Here's how the part is built. I have some questions about the finished solid (model axes, mm). A direction names the side the tool comes from. Give positions to 0.01 mm unless a question says otherwise; leave off trailing zeros. Write each loop counter-clockwise with the first axis right and the second up, starting at its lowest first coordinate (ties: lowest second). Pieces come first, ordered by that corner, then holes. Notation, with made-up numbers: (-11, 16) -> (33, 16) arc R25 ccw to (33, 44) -> close; hole circle Ø5 at (-20, 83). An arc over 180 degrees is marked (long way). Use one line per item in the form item = value.
```python
from build123d import *

# Parameters (mm, degrees)
BOSS_EXTRU_1_DEPTH       = 6
ESQUISSE4_W              = 107.5
ESQUISSE4_H              = 70
ENL_V_MAT_EXTRU_3_DEPTH  = 6
CONG_1_R                 = 20
CONG_2_R                 = 8
CONG_3_R                 = 3
ESQUISSE7_W              = 15
ESQUISSE7_H              = 3
ENL_V_MAT_EXTRU_6_DEPTH  = 10
ESQUISSE6_R              = 2
ENL_V_MAT_EXTRU_5_DEPTH  = 10
ESQUISSE8_R              = 2
ESQUISSE8_W              = 6
ESQUISSE8_H              = 12
ENL_V_MAT_EXTRU_7_DEPTH  = 10
ESQUISSE9_R              = 2
ESQUISSE9_W              = 6
ESQUISSE9_H              = 6
ENL_V_MAT_EXTRU_8_DEPTH  = 10
ESQUISSE10_W             = 15
ESQUISSE10_H             = 3
ENL_V_MAT_EXTRU_9_DEPTH  = 10
ESQUISSE11_R             = 1.5
ESQUISSE11_R_2           = 2
ESQUISSE11_R_3           = 1
ESQUISSE11_W             = 10
ESQUISSE11_H             = 6
ENL_V_MAT_EXTRU_10_DEPTH = 10


with BuildPart() as part:
    # Esquisse1 → Boss.-Extru.1 (new body)
    with BuildSketch(Plane(origin=(0, 0, 0), x_dir=(1, 0, 0), z_dir=(0, 1, 0))):
        with BuildLine():
            Line((-159.651418776, 61.996478628), (-151.00295557, 16.28223991))
            ThreePointArc((-151.00295557, 16.28223991), (-144.111724845, 4.599428553), (-131.351536794, 0))
            Line((-131.351536794, 0), (-50.176822125, 0))
            ThreePointArc((-50.176822125, 0), (0, -8.568957982), (50.176822125, 0))
            Line((50.176822125, 0), (131.351536794, 0))
            ThreePointArc((131.351536794, 0), (144.111724845, 4.599428553), (151.00295557, 16.28223991))
            Line((151.00295557, 16.28223991), (159.651418776, 61.996478628))
            ThreePointArc((159.651418776, 61.996478628), (159.912664005, 63.847205713), (160, 65.714238717))
            Line((160, 65.714238717), (160, 154.285761283))
            ThreePointArc((160, 154.285761283), (158.521020838, 161.833727042), (154.30282129, 168.265364394))
            Line((154.30282129, 168.265364394), (109.621642599, 213.979603112))
            ThreePointArc((109.621642599, 213.979603112), (103.077942966, 218.433557202), (95.31882131, 220))
            Line((95.31882131, 220), (-95.31882131, 220))
            ThreePointArc((-95.31882131, 220), (-103.077942966, 218.433557202), (-109.621642599, 213.979603112))
            Line((-109.621642599, 213.979603112), (-154.30282129, 168.265364394))
            ThreePointArc((-154.30282129, 168.265364394), (-158.521020838, 161.833727042), (-160, 154.285761283))
            Line((-160, 154.285761283), (-160, 65.714238717))
            ThreePointArc((-160, 65.714238717), (-159.912664005, 63.847205713), (-159.651418776, 61.996478628))
        make_face()
    extrude(amount=BOSS_EXTRU_1_DEPTH)

    # Esquisse4 → Enlèv. mat.-Extru.3 (cut)
    with BuildSketch(Plane(origin=(0, 6, 0), x_dir=(1, 0, 0), z_dir=(0, 1, 0))):
        with Locations((-98.75, 31)):
            Rectangle(ESQUISSE4_W, ESQUISSE4_H)
        with Locations((98.75, 31)):
            Rectangle(ESQUISSE4_W, ESQUISSE4_H)
    extrude(amount=-ENL_V_MAT_EXTRU_3_DEPTH, mode=Mode.SUBTRACT)

    # Congé1
    cong_1_edges = [part.edges().sort_by_distance(p)[0] for p in [
        (-45, 3, 1.716975434),
        (45, 3, 1.716975434),
    ]]
    fillet(cong_1_edges, radius=CONG_1_R)

    # Congé2
    cong_2_edges = [part.edges().sort_by_distance(p)[0] for p in [
        (-45, 3, -66),
        (-152.5, 3, -66),
        (152.5, 3, -66),
        (45, 3, -66),
    ]]
    fillet(cong_2_edges, radius=CONG_2_R)

    # Congé3
    cong_3_edges = [part.edges().sort_by_distance(p)[0] for p in [
        (-152.5, 3, -24.195350576),
        (152.5, 3, -24.195350576),
    ]]
    fillet(cong_3_edges, radius=CONG_3_R)

    # Esquisse7 → Enlèv. mat.-Extru.6 (cut)
    with BuildSketch(Plane(origin=(0, 6, 0), x_dir=(1, 0, 0), z_dir=(0, 1, 0))):
        with Locations((-25, 67.499999998)):
            Rectangle(ESQUISSE7_W, ESQUISSE7_H)
        with Locations((25, 67.499999998)):
            Rectangle(ESQUISSE7_W, ESQUISSE7_H)
    extrude(amount=-ENL_V_MAT_EXTRU_6_DEPTH, mode=Mode.SUBTRACT)

    # Esquisse6 → Enlèv. mat.-Extru.5 (cut)
    with BuildSketch(Plane(origin=(0, 6, 0), x_dir=(1, 0, 0), z_dir=(0, 1, 0))):
        with Locations(Location((0, 210, 0), (0, 0, 270))):
            Circle(ESQUISSE6_R)
    extrude(amount=-ENL_V_MAT_EXTRU_5_DEPTH, mode=Mode.SUBTRACT)

    # Esquisse8 → Enlèv. mat.-Extru.7 (cut)
    with BuildSketch(Plane(origin=(0, 6, 0), x_dir=(1, 0, 0), z_dir=(0, 1, 0))):
        with Locations(Location((-89.9, 110, 0), (0, 0, 270))):
            Circle(ESQUISSE8_R)
        with Locations(Location((-68.76, 110, 0), (0, 0, 270))):
            Circle(ESQUISSE8_R)
        with Locations(Location((-41.76, 110, 0), (0, 0, 270))):
            Circle(ESQUISSE8_R)
        with Locations(Location((41.76, 110, 0), (0, 0, 270))):
            Circle(ESQUISSE8_R)
        with Locations(Location((68.76, 110, 0), (0, 0, 270))):
            Circle(ESQUISSE8_R)
        with Locations(Location((89.9, 110, 0), (0, 0, 270))):
            Circle(ESQUISSE8_R)
        with Locations((-89.9, 96)):
            Rectangle(ESQUISSE8_W, ESQUISSE8_H)
        with Locations((-89.9, 124)):
            Rectangle(ESQUISSE8_W, ESQUISSE8_H)
        with Locations((-68.76, 96)):
            Rectangle(ESQUISSE8_W, ESQUISSE8_H)
        with Locations((-68.76, 124)):
            Rectangle(ESQUISSE8_W, ESQUISSE8_H)
        with Locations((-41.76, 96)):
            Rectangle(ESQUISSE8_W, ESQUISSE8_H)
        with Locations((-41.76, 124)):
            Rectangle(ESQUISSE8_W, ESQUISSE8_H)
        with Locations((41.76, 96)):
            Rectangle(ESQUISSE8_W, ESQUISSE8_H)
        with Locations((41.76, 124)):
            Rectangle(ESQUISSE8_W, ESQUISSE8_H)
        with Locations((68.76, 96)):
            Rectangle(ESQUISSE8_W, ESQUISSE8_H)
        with Locations((68.76, 124)):
            Rectangle(ESQUISSE8_W, ESQUISSE8_H)
        with Locations((89.9, 96)):
            Rectangle(ESQUISSE8_W, ESQUISSE8_H)
        with Locations((89.9, 124)):
            Rectangle(ESQUISSE8_W, ESQUISSE8_H)
    extrude(amount=-ENL_V_MAT_EXTRU_7_DEPTH, mode=Mode.SUBTRACT)

    # Esquisse9 → Enlèv. mat.-Extru.8 (cut)
    with BuildSketch(Plane(origin=(0, 6, 0), x_dir=(1, 0, 0), z_dir=(0, 1, 0))):
        with Locations(Location((147, 118.4, 0), (0, 0, 270))):
            Circle(ESQUISSE9_R)
        with Locations(Location((147, 87.4, 0), (0, 0, 270))):
            Circle(ESQUISSE9_R)
        with Locations((154, 118.4)):
            Rectangle(ESQUISSE9_W, ESQUISSE9_H)
        with Locations((154, 87.4)):
            Rectangle(ESQUISSE9_W, ESQUISSE9_H)
        with Locations((140, 118.4)):
            Rectangle(ESQUISSE9_W, ESQUISSE9_H)
        with Locations((140, 87.4)):
            Rectangle(ESQUISSE9_W, ESQUISSE9_H)
    extrude(amount=-ENL_V_MAT_EXTRU_8_DEPTH, mode=Mode.SUBTRACT)

    # Esquisse10 → Enlèv. mat.-Extru.9 (cut)
    with BuildSketch(Plane(origin=(0, 6, 0), x_dir=(1, 0, 0), z_dir=(0, 1, 0))):
        with Locations((-25, 176.83)):
            Rectangle(ESQUISSE10_W, ESQUISSE10_H)
        with Locations((25, 176.83)):
            Rectangle(ESQUISSE10_W, ESQUISSE10_H)
    extrude(amount=-ENL_V_MAT_EXTRU_9_DEPTH, mode=Mode.SUBTRACT)

    # Esquisse11 → Enlèv. mat.-Extru.10 (cut)
    with BuildSketch(Plane(origin=(0, 6, 0), x_dir=(-1, 0, 0), z_dir=(0, 1, 0))):
        with Locations(Location((40, -23.835046453, 0), (0, 0, 90))):
            Circle(ESQUISSE11_R)
        with Locations(Location((-40, -23.835046453, 0), (0, 0, 90))):
            Circle(ESQUISSE11_R)
        with Locations(Location((100.750206469, -212.903490041, 0), (0, 0, 90))):
            Circle(ESQUISSE11_R)
        with Locations(Location((152.964714587, -159.569337314, 0), (0, 0, 90))):
            Circle(ESQUISSE11_R)
        with Locations(Location((50.375103235, -212.903490041, 0), (0, 0, 90))):
            Circle(ESQUISSE11_R)
        with Locations(Location((-152.964714587, -159.569337314, 0), (0, 0, 90))):
            Circle(ESQUISSE11_R)
        with Locations(Location((-100.750206469, -212.903490041, 0), (0, 0, 90))):
            Circle(ESQUISSE11_R)
        with Locations(Location((-50.375103235, -212.903490041, 0), (0, 0, 90))):
            Circle(ESQUISSE11_R)
        with Locations(Location((0, -44.911042018, 0), (0, 0, 90))):
            Circle(ESQUISSE11_R)
        with Locations(Location((-109.47882131, -189.64, 0), (0, 0, 90))):
            Circle(ESQUISSE11_R_2)
        with Locations(Location((109.47882131, -189.64, 0), (0, 0, 90))):
            Circle(ESQUISSE11_R_2)
        with Locations(Location((142, -99.324238717, 0), (0, 0, 90))):
            Circle(ESQUISSE11_R_3)
        with Locations(Location((126, -99.324238717, 0), (0, 0, 90))):
            Circle(ESQUISSE11_R_3)
        with Locations(Location((126, -115.324238717, 0), (0, 0, 90))):
            Circle(ESQUISSE11_R_3)
        with Locations(Location((142, -115.324238717, 0), (0, 0, 90))):
            Circle(ESQUISSE11_R_3)
        with Locations((155, -130.324238717)):
            Rectangle(ESQUISSE11_W, ESQUISSE11_H)
        with Locations((155, -83.324238717)):
            Rectangle(ESQUISSE11_W, ESQUISSE11_H)
    extrude(amount=-ENL_V_MAT_EXTRU_10_DEPTH, mode=Mode.SUBTRACT)


solid = part.part
```
Q1. I want a section at C-C, the plane x = 125. Write out the boundary of the cut face in (y, z), and give its area (3 significant figures).
Result set:
outline = (0, -198.25) -> (6, -198.25) -> (6, -66) -> (0, -66) -> close
area = 793 mm2
Q2. I want a section at A-A, the plane z = -17.5. Write out the boundary of the cut face in (x, y).
Result set:
outline = (-45, 0) -> (45, 0) -> (45, 6) -> (-45, 6) -> close
Q3. Will these pins go through, and if not, where does the flat tip stop? pin 1 Ø1.5 at (y, z) = (2, -176.5) entering from +X; pin 2 Ø2.5 at (x, z) = (40, -23.84) entering from +Y; pin 3 Ø0.5 at (y, z) = (3, -57.5) entering from +X; pin 4 Ø3 at (x, y) = (-67.5, 1.5) entering from +Z.
Result set:
pin_1 = 146.99
pin_2 = through
pin_3 = 158.85
pin_4 = -66
Q4. I want a section at B-B, the plane y = 4.5. Count the separate pieces of the cut face and the enclosed holes in it, and give its area (3 significant figures).
Result set:
separate_pieces = 1
enclosed_holes = 44
area = 51,100 mm2
Q5. Which directions (+Z, -Z, +X, -X, +Y, -Y) give clear straight access to the entire face, cutting with the end or side of a thin tool? Please do faces 1 (the face through (-99, 3, -66)), 2 (the face through (-155, 3, -86.324)), 3 (the face through (159.04, 2.96, -58.77)), 4 (the face through (-69, 3, -102)), 5 (the face through (-160, 3, -144)).
Result set:
face_1 = +Z, +Y, -Y
face_2 = -X, +Y, -Y
face_3 = +Z, +X, +Y, -Y
face_4 = +Y, -Y
face_5 = +Z, -Z, -X, +Y, -Y
Q6. If I drill on line 1 along Z through (x, y) = (69, 1.5); line 2 along Z through (x, y) = (-125.5, 3.15); line 3 along X through (y, z) = (4.55, -87.4), over which ranges is the centre line in solid material (lowest first)? Write a range as from..to.
Result set:
line_1 = -220..-130, -118..-111.99, -108.01..-102, -90..-66
line_2 = -197.73..-116.19, -114.46..-100.19, -98.46..-66
line_3 = -160..137, 143..145, 149..151, 157..160
